```python
from build123d import *

# Parameters (mm, degrees)
SKETCH1_W           = 58
SKETCH1_H           = 24
SKETCH1_R           = 2.1
SKETCH1_W_2         = 40.4
SKETCH1_H_2         = 21.3
BOSS_EXTRUDE1_DEPTH = 28.35
SKETCH11_W          = 58
SKETCH11_H          = 24
BOSS_EXTRUDE5_DEPTH = 3.175
SKETCH14_W          = 24
SKETCH14_H          = 12
BOSS_EXTRUDE7_DEPTH = 9
CUT_EXTRUDE1_START  = -4.5
CUT_EXTRUDE1_DEPTH  = 7.6
FILLET1_R           = 8
CHAMFER2_SIZE       = 3
CHAMFER3_SIZE       = 1
SKETCH19_W          = 8
SKETCH19_H          = 6
CUT_EXTRUDE3_DEPTH  = 2.75
SKETCH20_W          = 8.8
SKETCH20_H          = 8.5
CUT_EXTRUDE4_DEPTH  = 4
SKETCH21_W          = 20
SKETCH21_H          = 20
BOSS_EXTRUDE8_DEPTH = 6
SKETCH13_R          = 2.55
BOSS_EXTRUDE6_DEPTH = 5
FILLET4_R           = 1
CHAMFER4_SIZE       = 2
FILLET5_R           = 1
CUT_EXTRUDE5_REACH  = 77.835
SKETCH22_W          = 7
SKETCH22_H          = 7
CUT_EXTRUDE6_DEPTH  = 1.4
SKETCH24_R          = 3.125
CUT_EXTRUDE7_DEPTH  = 1.35


with BuildPart() as part:
    # Sketch1 → Boss-Extrude1 (new body)
    with BuildSketch(Plane(origin=(0, 0, 0), x_dir=(1, 0, 0), z_dir=(0, 1, 0))):
        with Locations((29.95, -9.622651473)):
            Rectangle(SKETCH1_W, SKETCH1_H)
        with Locations(Location((55.15, -4.622651473, 0), (0, 0, 270))):
            Circle(SKETCH1_R, mode=Mode.SUBTRACT)
        with Locations(Location((55.15, -14.622651473, 0), (0, 0, 270))):
            Circle(SKETCH1_R, mode=Mode.SUBTRACT)
        with Locations(Location((4.75, -14.622651473, 0), (0, 0, 90))):
            Circle(SKETCH1_R, mode=Mode.SUBTRACT)
        with Locations(Location((4.75, -4.622651473, 0), (0, 0, 90))):
            Circle(SKETCH1_R, mode=Mode.SUBTRACT)
        with Locations((29.95, -9.622651473)):
            Rectangle(SKETCH1_W_2, SKETCH1_H_2, mode=Mode.SUBTRACT)
    extrude(amount=BOSS_EXTRUDE1_DEPTH)

    # Sketch11 → Boss-Extrude5 (add)
    with BuildSketch(Plane.XZ):
        with Locations((29.95, 9.622651473)):
            Rectangle(SKETCH11_W, SKETCH11_H)
    extrude(amount=BOSS_EXTRUDE5_DEPTH)

    # Sketch14 → Boss-Extrude7 (add)
    with BuildSketch(Plane(origin=(0, 0, -2.377348527), x_dir=(-1, 0, 0), z_dir=(0, 0, -1))):
        with Locations((-12.95, 12.5875)):
            Rectangle(SKETCH14_W, SKETCH14_H)
    extrude(amount=BOSS_EXTRUDE7_DEPTH)

    # Sketch16 → Cut-Extrude1 (cut)
    with BuildSketch(Plane(origin=(0, 0, -6.877348527), x_dir=(-1, 0, 0), z_dir=(0, 0, -1)).offset(CUT_EXTRUDE1_START)):
        with BuildLine():
            Line((-11.45, 16.7875), (-24.95, 16.7875))
            Line((-24.95, 16.7875), (-24.95, 8.3875))
            Line((-24.95, 8.3875), (-11.45, 8.3875))
            ThreePointArc((-11.45, 8.3875), (-7.25, 12.5875), (-11.45, 16.7875))
        make_face()
    extrude(amount=CUT_EXTRUDE1_DEPTH, mode=Mode.SUBTRACT)

    # Fillet1
    fillet1_edges = [part.edges().sort_by_distance(p)[0] for p in [
        (12.95, 6.5875, -2.377348527),
        (12.95, 18.5875, -2.377348527),
    ]]
    fillet(fillet1_edges, radius=FILLET1_R)

    # Chamfer2
    chamfer2_edges = [part.edges().sort_by_distance(p)[0] for p in [
        (0.95, 6.5875, -10.877348527),
        (0.95, 18.5875, -10.877348527),
        (58.95, 12.5875, 21.622651473),
        (0.95, 12.5875, 21.622651473),
        (0.95, 27.46875, -2.377348527),
        (58.95, 12.5875, -2.377348527),
        (0.95, -2.29375, -2.377348527),
        (0.95, 4.244354249, -4.720494277),
        (0.95, 20.930645751, -4.720494277),
    ]]
    chamfer(chamfer2_edges, length=CHAMFER2_SIZE)

    # Chamfer3
    chamfer3_edges = [part.edges().sort_by_distance(p)[0] for p in [
        (14.45, 6.5875, -11.377348527),
        (24.95, 12.5875, -11.377348527),
        (14.45, 18.5875, -11.377348527),
        (0.95, 12.5875, -11.377348527),
    ]]
    chamfer(chamfer3_edges, length=CHAMFER3_SIZE - 0.0001)  # a hair under: the kernel refuses the full size

    # Sketch19 → Cut-Extrude3 (cut)
    with BuildSketch(Plane(origin=(0, 25.35, 0), x_dir=(1, 0, 0), z_dir=(0, 1, 0))):
        with Locations((4.95, -4.622651473)):
            Rectangle(SKETCH19_W, SKETCH19_H)
        with Locations((4.95, -14.622651473)):
            Rectangle(SKETCH19_W, SKETCH19_H)
        with Locations((54.95, -14.622651473)):
            Rectangle(SKETCH19_W, SKETCH19_H)
        with Locations((54.95, -4.622651473)):
            Rectangle(SKETCH19_W, SKETCH19_H)
    extrude(amount=-CUT_EXTRUDE3_DEPTH, mode=Mode.SUBTRACT)

    # Sketch20 → Cut-Extrude4 (cut)
    with BuildSketch(Plane(origin=(0, 0, 0), x_dir=(1, 0, 0), z_dir=(0, 1, 0))):
        with Locations((5.35, -9.622651473)):
            Rectangle(SKETCH20_W, SKETCH20_H)
    extrude(amount=CUT_EXTRUDE4_DEPTH, mode=Mode.SUBTRACT)

    # Sketch21 → Boss-Extrude8 (add)
    with BuildSketch(Plane.XZ.offset(3.175)):
        with Locations((20, 9.622651473)):
            Rectangle(SKETCH21_W, SKETCH21_H)
    extrude(amount=BOSS_EXTRUDE8_DEPTH)

    # Sketch13 → Boss-Extrude6 (add)
    with BuildSketch(Plane.XZ.offset(9.175)):
        with Locations(Location((20, 9.622651473, 0), (0, 0, 270))):
            Circle(SKETCH13_R)
    extrude(amount=BOSS_EXTRUDE6_DEPTH)

    # Fillet4
    fillet4_edges = [part.edges().sort_by_distance(p)[0] for p in [
        (10, -3.175, 9.622651473),
        (20, -3.175, -0.377348527),
        (30, -3.175, 9.622651473),
        (20, -3.175, 19.622651473),
    ]]
    fillet(fillet4_edges, radius=FILLET4_R)

    # Chamfer4
    chamfer4_edges = [part.edges().sort_by_distance(p)[0] for p in [
        (10, -9.175, 9.622651473),
        (20, -9.175, -0.377348527),
        (30, -9.175, 9.622651473),
        (20, -9.175, 19.622651473),
    ]]
    chamfer(chamfer4_edges, length=CHAMFER4_SIZE)

    # Fillet5
    fillet5_edges = [part.edges().sort_by_distance(p)[0] for p in [
        (20, -14.175, 12.172651473),
    ]]
    fillet(fillet5_edges, radius=FILLET5_R)

    # Cut-Extrude5: up to this face of the body (flat: up to its plane)
    cut_extrude5_end = Plane(part.part.faces().sort_by_distance((27.49586415, 0, 9.622651473))[0])
    # Sketch22 → Cut-Extrude5 (cut, up to the picked face)
    with BuildSketch(Plane(origin=(0, 28.35, 0), x_dir=(1, 0, 0), z_dir=(0, 1, 0)), mode=Mode.PRIVATE) as cut_extrude5_sk1:
        with Locations((6.25, -9.622651473)):
            Rectangle(SKETCH22_W, SKETCH22_H)
    cut_extrude5_tool1 = split(extrude(cut_extrude5_sk1.sketch, amount=-CUT_EXTRUDE5_REACH, mode=Mode.PRIVATE), bisect_by=cut_extrude5_end, keep=Keep.BOTH, mode=Mode.PRIVATE)
    add(cut_extrude5_tool1.solids().sort_by(Axis((6.25, 28.35, 9.622651), (0, -1, 0)))[0], mode=Mode.SUBTRACT)

    # Sketch23 → Cut-Extrude6 (cut)
    with BuildSketch(Plane(origin=(0, 0, -11.377348527), x_dir=(-1, 0, 0), z_dir=(0, 0, -1))):
        with BuildLine():
            ThreePointArc((-10.2, 12.5875), (-11.45, 13.8375), (-12.7, 12.5875))
            ThreePointArc((-12.7, 12.5875), (-11.45, 11.3375), (-10.2, 12.5875))
        make_face()
        with BuildLine():
            ThreePointArc((-14.2, 12.5875), (-15.45, 13.8375), (-16.7, 12.5875))
            ThreePointArc((-16.7, 12.5875), (-15.45, 11.3375), (-14.2, 12.5875))
        make_face()
    extrude(amount=-CUT_EXTRUDE6_DEPTH, mode=Mode.SUBTRACT)

    # Sketch24 → Cut-Extrude7 (cut)
    with BuildSketch(Plane(origin=(0, 0, -2.377348527), x_dir=(-1, 0, 0), z_dir=(0, 0, -1))):
        with Locations((-35.45, 12.5875)):
            Circle(SKETCH24_R)
    extrude(amount=-CUT_EXTRUDE7_DEPTH, mode=Mode.SUBTRACT)


solid = part.part
```
Check sheet for the modelled part. Datum: model origin and axes. Units: mm. A direction names the side the tool comes from. Give positions to 0.01 mm unless a question says otherwise; leave off trailing zeros. Loops run counter-clockwise (first coordinate to the right, second up) from the corner with the lowest first, then second, coordinate; pieces in that order, holes last. Notation, with made-up numbers: M 78,48 L 92,48 A29 ccw 92,77 Z; hole C -27.75,47 d8. An arc over 180 degrees is marked long. Answer as CSV lines item,"result".
Item 1: Sectioned sample at D-D, the plane y = -10. Enter the section's corners in (x, z).
Reply:
outline,"C 20,9.62 d5.1"
Item 2: Sectioned sample at C-C, the plane x = 47. Enter the section's corners in (y, z) (3 decimals), then the cut area to 3 significant figures.
Reply:
outline,"M -3.175,-2.377 L 28.35,-2.377 L 28.35,-1.027 L 0,-1.027 L 0,20.273 L 28.35,20.273 L 28.35,21.623 L -3.175,21.623 Z"
area,"153 mm^2"
Item 3: Depth check by flat-ended pin: pin 1 Ø0.8 at (x, y) = (54.5, 24) entering from -Z; pin 2 Ø1.8 at (x, z) = (6.5, 3.5) entering from -Y (3 decimals); pin 3 Ø2 at (y, z) = (19, -7) entering from +X. Enter the tip coordinate at first touch or a pass-through.
Reply:
pin 1,"z = -2.38"
pin 2,"y = -3.175"
pin 3,"x = 24.95"
Item 4: Draft check along X on faces 1 (the face through (25, 0, 9)), 2 (the face through (58.95, 13, 9)), 3 (the face through (9.75, 14, 17)), 4 (the face through (55, 24, 17.623)). Enter one of: pulls with the +X half, pulls with the -X half, needs draft (parallel to the pull), parting line crosses it, or undercut.
Reply:
face 1,"undercut"
face 2,"pulls with the +X half"
face 3,"undercut"
face 4,"needs draft"
Item 5: Set-up check for faces 5 (the face through (24.95, 8, -5)), 6 (the face through (2.75, 16, 10)), 7 (the face through (55, 24, 1.623)), 8 (the face through (8, 2, 5.373)): record each of +Z, -Z, +X, -X, +Y, -Y from which the full face is reachable in a straight line by a thin tool's end or side.
Reply:
face 5,"-Z, +X, +Y, -Y"
face 6,"+Y"
face 7,"+X"
face 8,"-X"
Item 6: Scan lines: L1, parallel to Z at x = 55.15, y = 10.75; L2, parallel to Z at x = 21.5, y = 12; L3, parallel to Z at x = 29.5, y = 26. Record each from-to range of solid material in increasing order.
Reply:
L1,"-2.38 to 2.52, 6.72 to 12.52, 16.72 to 21.62"
L2,"-11.38 to -9.98, -2.38 to -1.03, 20.27 to 21.62"
L3,"-2.38 to -1.03, 20.27 to 21.62"
